Design review of the part shown in the three views and the two pictorial views. Dimensions are in mm from the part's minimum x, y and z. Coordinates: 2 decimals unless noted, no trailing zeros. Loops run counter-clockwise (first coordinate to the right, second up) from the corner with the lowest first, then second, coordinate; pieces in that order, holes last. Notation, with made-up numbers: M 9.5,7.25 L 43.5,7.25 A34 ccw 43.5,37.25 Z; hole C 9,17 d2. An arc over 180 degrees is marked long. Answer as a JSON object with one key per item and string values. Group by question number.
Item 1: Add section A-A (y = 22.86). State the section outline as (x, z) points.
Item 2: Add section D-D (x = 295). State the section outline as (y, z) points.
Item 3: Add section B-B (z = 1.75). State the section outline as (x, y) points.
Item 4: Add section C-C (x = 355.6). State the section outline as (y, z) points.
Item 5: Wall thickness on L1, parallel to Y at x = 355.6, z = 1.5; L2, parallel to Y at x = 362, z = 4; L3, parallel to X at y = 36, z = 5: over which ranges is each line inside the solid? List them lowest first. Write a range as from..to.
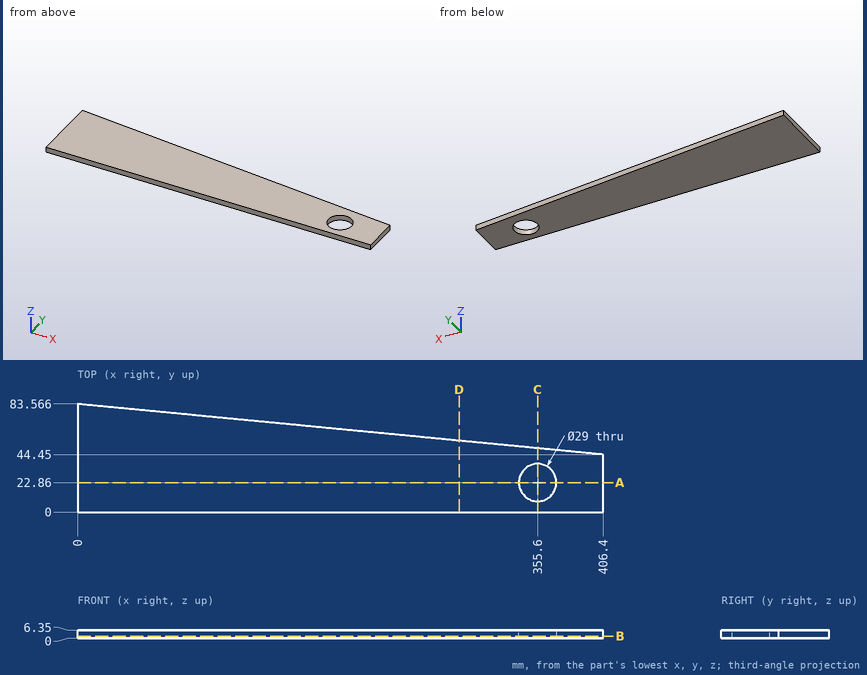
From the geometry:
{
 "1": {"outline": "M 0,0 L 341.1,0 L 341.1,6.35 L 0,6.35 Z; M 370.1,0 L 406.4,0 L 406.4,6.35 L 370.1,6.35 Z"},
 "2": {"outline": "M 0,0 L 55.17,0 L 55.17,6.35 L 0,6.35 Z"},
 "3": {"outline": "M 0,0 L 406.4,0 L 406.4,44.45 L 0,83.57 Z; hole C 355.6,22.86 d29"},
 "4": {"outline": "M 0,0 L 8.36,0 L 8.36,6.35 L 0,6.35 Z; M 37.36,0 L 49.34,0 L 49.34,6.35 L 37.36,6.35 Z"},
 "5": {"L1": "y = 0..8.36, 37.36..49.34", "L2": "y = 0..9.85, 35.87..48.72", "L3": "x = 0..349.47, 361.73..406.4"}
}
